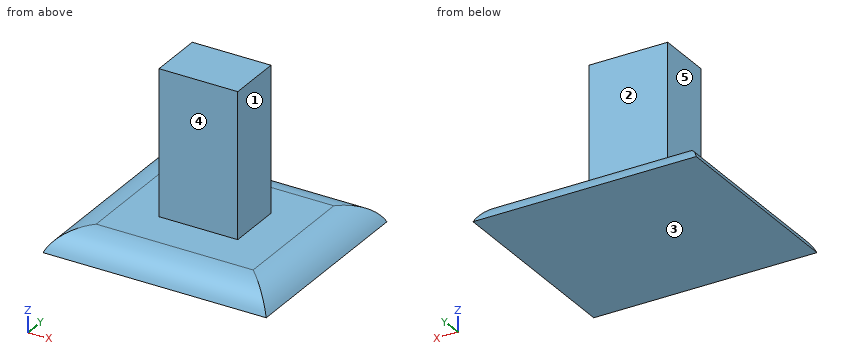
from build123d import *

# Parameters (mm, degrees)
F0_W        = 10.9
F0_H        = 7.6
F1_DEPTH    = 20
F2_W        = 30.9
F2_H        = 27.6
F2_W_2      = 10.9
F2_H_2      = 7.6
F3_DEPTH    = 3
F4_T1_DEPTH = 50.5128784748
F4_T3_DEPTH = 53.8128784748


# Not quite as in the source:
# - a fillet or chamfer that OpenCascade refuses, or shapes differently, is made with other operations: its cross-section is extruded or revolved along the edge and cut away or added


with BuildPart() as f1:
    # F0 (on Top) → F1 (new body)
    with BuildSketch(Plane.XY):
        with Locations((1.5206737995, 10.1067991287)):
            Rectangle(F0_W, F0_H)
    extrude(amount=F1_DEPTH)

    # F2 (on face) → F3 (join)
    with BuildSketch(Plane(origin=(0, 0, 0), x_dir=(1, 0, 0), z_dir=(0, 0, -1))):
        with Locations((1.5206737995, -10.1067991287)):
            Rectangle(F2_W, F2_H)
        with Locations((1.5206737995, -10.1067991287)):
            Rectangle(F2_W_2, F2_H_2, mode=Mode.SUBTRACT)
        with Locations((1.5206737995, -10.1067991287)):
            Rectangle(F2_W_2, F2_H_2)
    extrude(amount=F3_DEPTH)

    # F4: fillet of radius 5 on 4 edges, made by hand

    # F4_s2 → F4_t1 (cut)
    with BuildSketch(Plane.XZ.offset(-35.363238366)):
        with BuildLine():
            ThreePointArc((-13.9293262005, -3), (-12.0853632931, -0.8166998673), (-9.3467505055, 0))
            Line((-9.3467505055, 0), (-13.9293262005, 0))
            Line((-13.9293262005, 0), (-13.9293262005, -3))
        make_face()
        with BuildLine():
            ThreePointArc((12.3880981046, 0), (15.1267108921, -0.8166998673), (16.9706737995, -3))
            Line((16.9706737995, -3), (16.9706737995, 0))
            Line((16.9706737995, 0), (12.3880981046, 0))
        make_face()
    extrude(amount=F4_T1_DEPTH, mode=Mode.SUBTRACT)

    # F4_s4 → F4_t3 (cut)
    with BuildSketch(Plane.YZ.offset(-25.3857654379)):
        with BuildLine():
            ThreePointArc((-3.6932008713, -3), (-1.8492379639, -0.8166998673), (0.8893748236, 0))
            Line((0.8893748236, 0), (-3.6932008713, 0))
            Line((-3.6932008713, 0), (-3.6932008713, -3))
        make_face()
        with BuildLine():
            ThreePointArc((23.9067991287, -3), (22.0628362212, -0.8166998673), (19.3242234337, 0))
            Line((19.3242234337, 0), (23.9067991287, 0))
            Line((23.9067991287, 0), (23.9067991287, -3))
        make_face()
    extrude(amount=F4_T3_DEPTH, mode=Mode.SUBTRACT)


solid = f1.part
Design review of the part built by this model. Coordinates are the model's own, in mm. Face numbers are marked on the shaded views. A direction names the side the tool comes from. Give positions to 0.01 mm unless a question says otherwise; leave off trailing zeros. Order: outer loops, then holes, each group sorted by start corner. A loop starts at its lowest first (then second) coordinate and runs counter-clockwise, first axis right, second up. Notation, with made-up numbers: (-12.75, -30) - (32.25, -30) arc R29 ccw to (32.25, 7) - close; hole circle Ø5 at (88.25, 11). An arc over 180 degrees is marked (long way). Write item = value, one per line. Start each with the question number.
Q1. Clearance check with flat-ended pins moving along their axes: pin 1 Ø8.5 at (y, z) = (11, 10) entering from +X; pin 2 Ø5.5 at (x, z) = (4, 5) entering from +Y; pin 3 Ø10 at (y, z) = (20, 4.5) entering from -X. State where each tip first meets the part, or that it passes through.
Q2. To check wall thickness, follow L1, parallel to X at y = 7, z = 5.25; L2, parallel to Z at x = 1, y = 16.5; L3, parallel to Y at x = 3, z = 15.5. State the ranges of each line that lie inside material, in increasing order. Write a range as from..to.
Q3. We need section C-C on z = 7.75. State the section outline as (x, y) points, plus the area to 3 significant figures.
Q4. We need section A-A on y = 13.5. State the section outline as (x, z) points, plus the area to 3 significant figures.
Q5. We need section D-D on x = 11.5. State the section outline as (y, z) points.
Q6. Tool access review of the marked faces 1, 2, 3, 4 and 5: name each direction out of +Z, -Z, +X, -X, +Y, -Y from which nothing blocks a thin tool from reaching the whole face with its end or side.
Q7. We need section B-B on x = 2.5. State the section outline as (y, z) points, plus the area to 3 significant figures.
Working result:
q1.pin_1 = 6.97
q1.pin_2 = 13.91
q1.pin_3 = -11.53
q2.L1 = -3.93..6.97
q2.L2 = -3..0
q2.L3 = 6.31..13.91
q3.outline = (-3.93, 6.31) - (6.97, 6.31) - (6.97, 13.91) - (-3.93, 13.91) - close
q3.area = 82.8 mm²
q4.outline = (-13.93, -3) - (16.97, -3) arc R5 ccw to (12.39, 0) - (6.97, 0) - (6.97, 20) - (-3.93, 20) - (-3.93, 0) - (-9.35, 0) arc R5 ccw to start
q4.area = 303 mm²
q5.outline = (-3.69, -3) - (23.91, -3) arc R5 ccw to (19.32, 0) - (0.89, 0) arc R5 ccw to start
q6.face_1 = +Z, +X, +Y, -Y
q6.face_2 = +Z, +X, -X, +Y
q6.face_3 = -Z, +X, -X, +Y, -Y
q6.face_4 = +Z, +X, -X, -Y
q6.face_5 = +Z, -X, +Y, -Y
q7.outline = (-3.69, -3) - (23.91, -3) arc R5 ccw to (19.32, 0) - (13.91, 0) - (13.91, 20) - (6.31, 20) - (6.31, 0) - (0.89, 0) arc R5 ccw to start
q7.area = 227 mm²
